Geometry: final body of the model. Coordinates: model frame, mm. Face numbers are marked on the shaded views. A direction names the side the tool comes from. Round coordinates to 2 decimals unless told otherwise and drop trailing zeros. Loops run counter-clockwise (first coordinate to the right, second up) from the corner with the lowest first, then second, coordinate; pieces in that order, holes last. Notation, with made-up numbers: (14, 14) -> (38, 14) arc R14 ccw to (38, 20) -> close; hole circle Ø9 at (83.25, 45). An arc over 180 degrees is marked (long way). Answer in a Markdown table with one row per item.
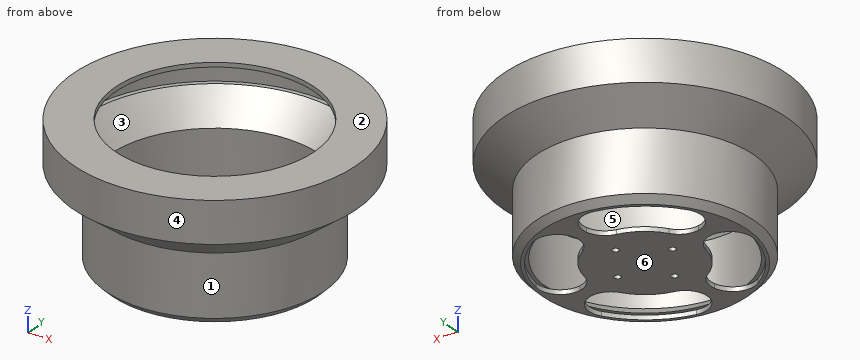
```python
from build123d import *

# Parameters (mm, degrees)
BOSS_EXTRUDE2_START = 2
SKETCH3_R           = 49.35
SKETCH3_R_2         = 1.5
BOSS_EXTRUDE2_DEPTH = 2
FILLET1_R           = 10
FILLET2_R           = 10
CHAMFER1_SIZE       = 3
SKETCH6_W           = 130.40409261
SKETCH6_H           = 9
CUT_EXTRUDE1_DEPTH  = 72
SKETCH7_R           = 64
SKETCH7_R_2         = 45
BOSS_EXTRUDE3_DEPTH = 2


with BuildPart() as part:
    # Sketch2 → Revolve1 (revolve)
    with BuildSketch(Plane(origin=(0, 0, 0), x_dir=(0, 0, -1), z_dir=(1, 0, 0)), mode=Mode.PRIVATE) as revolve1_sk:
        Polygon((65.6, 47.35), (37, 47.35), (36.023809561, 47.35), (24, 60), (24, 62), (0, 62), (0, 64), (25.567979838, 64), (37, 49.35), (65.6, 49.35), align=None)
    revolve(revolve1_sk.sketch.rotate(Axis((0, 0, 1), (0, 0, -1)), 90), axis=Axis((0, 0, 1), (0, 0, -1)))

    # Sketch3 → Boss-Extrude2 (add)
    with BuildSketch(Plane(origin=(0, 0, -65.6), x_dir=(-1, 0, 0), z_dir=(0, 0, -1)).offset(BOSS_EXTRUDE2_START)):
        with Locations(Location((0, 0, 0), (0, 0, 180))):
            Circle(SKETCH3_R)
        with Locations((-14.646406867, -3.237709975)):
            Circle(SKETCH3_R_2, mode=Mode.SUBTRACT)
        with Locations((-3.237709975, 14.646406867)):
            Circle(SKETCH3_R_2, mode=Mode.SUBTRACT)
        with Locations((3.237709975, -14.646406867)):
            Circle(SKETCH3_R_2, mode=Mode.SUBTRACT)
        with Locations((14.646406867, 3.237709975)):
            Circle(SKETCH3_R_2, mode=Mode.SUBTRACT)
        with BuildLine():
            Line((2.426668662, -24.876217196), (6.743615296, -44.404759685))
            ThreePointArc((6.743615296, -44.404759685), (-24.155488069, -37.865174318), (-43.109904177, -12.601527718))
            Line((-43.109904177, -12.601527718), (-23.581361687, -8.284581085))
            ThreePointArc((-23.581361687, -8.284581085), (-13.442501867, -21.071640807), (2.426668662, -24.876217196))
        make_face(mode=Mode.SUBTRACT)
        with BuildLine():
            Line((-24.876217196, -2.426668662), (-44.404759685, -6.743615296))
            ThreePointArc((-44.404759685, -6.743615296), (-37.865174318, 24.155488069), (-12.601527718, 43.109904177))
            Line((-12.601527718, 43.109904177), (-8.284581085, 23.581361687))
            ThreePointArc((-8.284581085, 23.581361687), (-21.071640807, 13.442501867), (-24.876217196, -2.426668662))
        make_face(mode=Mode.SUBTRACT)
        with BuildLine():
            Line((-2.426668662, 24.876217196), (-6.743615296, 44.404759685))
            ThreePointArc((-6.743615296, 44.404759685), (24.155488069, 37.865174318), (43.109904177, 12.601527718))
            Line((43.109904177, 12.601527718), (23.581361687, 8.284581085))
            ThreePointArc((23.581361687, 8.284581085), (13.442501867, 21.071640807), (-2.426668662, 24.876217196))
        make_face(mode=Mode.SUBTRACT)
        with BuildLine():
            Line((8.284581085, -23.581361687), (12.601527718, -43.109904177))
            ThreePointArc((12.601527718, -43.109904177), (37.865174318, -24.155488069), (44.404759685, 6.743615296))
            Line((44.404759685, 6.743615296), (24.876217196, 2.426668662))
            ThreePointArc((24.876217196, 2.426668662), (21.071640807, -13.442501867), (8.284581085, -23.581361687))
        make_face(mode=Mode.SUBTRACT)
    extrude(amount=-BOSS_EXTRUDE2_DEPTH)

    # Fillet1
    # the kernel refuses this fillet: 10 mm, written as the material it adds along each edge
    with BuildSketch(Plane(origin=(-12.601527718, -43.109904177, -67.6), x_dir=(-0.9040126559830293, 0.4275056933217488, 0), z_dir=(0, 0, 1))) as fillet1_piece_1:
        with BuildLine():
            CenterArc((12.508516939, -9.876472905), FILLET1_R, 80.98497739, 111.859148491)
            Line((2.758732525, -12.099467257), (0, 0))
            ThreePointArc((0, 0), (7.037725598, 0.554809366), (14.075451195, 0))
        make_face()
    extrude(amount=2)
    with BuildSketch(Plane(origin=(-8.284581085, -23.581361687, -67.6), x_dir=(-0.8924722154511289, 0.45110236604096154, 0), z_dir=(0, 0, 1))) as fillet1_piece_2:
        with BuildLine():
            CenterArc((7.785535121, 9.915423441), FILLET1_R, 194.349189504, 68.193723572)
            Line((-1.902498089, 7.437115043), (0, 0))
            ThreePointArc((0, 0), (3.243849617, 0.211393168), (6.487699233, 0))
        make_face()
    extrude(amount=2)
    with BuildSketch(Plane(origin=(-24.876217196, 2.426668662, -67.6), x_dir=(-0.9764271244734938, 0.21584733167779538, 0), z_dir=(0, 0, 1))) as fillet1_piece_3:
        with BuildLine():
            CenterArc((7.676408375, 10), FILLET1_R, 201.807483199, 68.192516801)
            ThreePointArc((-1.607964784, 6.285109014), (-0.599195502, 3.194946614), (0, 0))
            Line((0, 0), (7.676408375, 0))
        make_face()
    extrude(amount=2)
    with BuildSketch(Plane(origin=(-44.404759685, 6.743615296, -67.6), x_dir=(0.006629845184633897, -0.999978022334905, 0), z_dir=(0, 0, 1))) as fillet1_piece_4:
        with BuildLine():
            CenterArc((12.508734152, 9.876468588), FILLET1_R, 167.15489194, 111.860288522)
            Line((2.758987847, 12.099630073), (0, 0))
            ThreePointArc((0, 0), (7.037847809, -0.554828755), (14.075695618, 0))
        make_face()
    extrude(amount=2)

    # Fillet2
    # the kernel refuses this fillet: 10 mm, written as the material it adds along each edge
    with BuildSketch(Plane(origin=(-43.109904177, 12.601527718, -67.6), x_dir=(0.4275056933217496, 0.9040126559830289, 0), z_dir=(0, 0, 1))) as fillet2_piece_1:
        with BuildLine():
            CenterArc((12.508516939, -9.876472905), FILLET2_R, 80.98497739, 111.859148491)
            Line((2.758732525, -12.099467257), (0, 0))
            ThreePointArc((0, 0), (7.037725598, 0.554809366), (14.075451195, 0))
        make_face()
    extrude(amount=2)
    with BuildSketch(Plane(origin=(-23.581361687, 8.284581085, -67.6), x_dir=(-0.9764271244734907, 0.21584733167780967, 0), z_dir=(0, 0, 1)), Plane(origin=(8.284581085, 23.581361687, -67.6), x_dir=(0.21584733167780917, 0.9764271244734908, 0), z_dir=(0, 0, 1)), Plane(origin=(23.581361687, -8.284581085, -67.6), x_dir=(0.9764271244734907, -0.21584733167780934, 0), z_dir=(0, 0, 1))) as fillet2_piece_2:
        with BuildLine():
            CenterArc((7.676599451, -10), FILLET2_R, 90, 68.193723572)
            ThreePointArc((-1.607851949, -6.285304563), (-0.599127572, -3.195042028), (0, 0))
            Line((0, 0), (7.676599451, 0))
        make_face()
    extrude(amount=2)
    with BuildSketch(Plane(origin=(2.426668662, 24.876217196, -67.6), x_dir=(0.2158473316777956, 0.9764271244734938, 0), z_dir=(0, 0, 1))) as fillet2_piece_3:
        with BuildLine():
            CenterArc((7.676408375, 10), FILLET2_R, 201.807483199, 68.192516801)
            ThreePointArc((-1.607964784, 6.285109014), (-0.599195502, 3.194946614), (0, 0))
            Line((0, 0), (7.676408375, 0))
        make_face()
    extrude(amount=2)
    with BuildSketch(Plane(origin=(6.743615296, 44.404759685, -67.6), x_dir=(-0.999978022334905, -0.006629845184635393, 0), z_dir=(0, 0, 1)), Plane(origin=(44.404759685, -6.743615296, -67.6), x_dir=(-0.006629845184635893, 0.999978022334905, 0), z_dir=(0, 0, 1)), Plane(origin=(-6.743615296, -44.404759685, -67.6), x_dir=(0.999978022334905, 0.00662984518463539, 0), z_dir=(0, 0, 1))) as fillet2_piece_4:
        with BuildLine():
            CenterArc((12.508734152, 9.876468588), FILLET2_R, 167.15489194, 111.860288522)
            Line((2.758987847, 12.099630073), (0, 0))
            ThreePointArc((0, 0), (7.037847809, -0.554828755), (14.075695618, 0))
        make_face()
    extrude(amount=2)
    with BuildSketch(Plane(origin=(24.876217196, -2.426668662, -67.6), x_dir=(-0.032899449429987265, 0.9994586665926729, 0), z_dir=(0, 0, 1)), Plane(origin=(-2.426668662, -24.876217196, -67.6), x_dir=(0.9994586665926729, 0.03289944942998876, 0), z_dir=(0, 0, 1))) as fillet2_piece_5:
        with BuildLine():
            CenterArc((7.785341334, -9.915427669), FILLET2_R, 97.456900257, 68.192516801)
            Line((-1.902631601, -7.436883658), (0, 0))
            ThreePointArc((0, 0), (3.243768875, -0.2113826), (6.48753775, 0))
        make_face()
    extrude(amount=2)
    with BuildSketch(Plane(origin=(12.601527718, 43.109904177, -67.6), x_dir=(-0.21584733167780898, -0.9764271244734908, 0), z_dir=(0, 0, 1)), Plane(origin=(43.109904177, -12.601527718, -67.6), x_dir=(-0.9764271244734909, 0.21584733167780892, 0), z_dir=(0, 0, 1))) as fillet2_piece_6:
        with BuildLine():
            CenterArc((12.40998441, 10), FILLET2_R, 158.140851509, 111.859148491)
            ThreePointArc((3.128964851, 13.723261468), (1.023555255, 6.984964542), (0, 0))
            Line((0, 0), (12.40998441, 0))
        make_face()
    extrude(amount=2)

    # Sketch5 → Revolve2 (revolve)
    with BuildSketch(Plane(origin=(0, 0, 0), x_dir=(1, 0, 0), z_dir=(0, 1, 0)), mode=Mode.PRIVATE) as revolve2_sk:
        Polygon((-47.35, 61.6), (-43.35, 65.6), (-47.35, 65.6), align=None)
    revolve(revolve2_sk.sketch.rotate(Axis((0, 0, 0), (0, 0, -1)), 180), axis=Axis((0, 0, 0), (0, 0, -1)))

    # Chamfer1
    chamfer1_edges = [part.edges().sort_by_distance(p)[0] for p in [
        (-49.35, 0, -67.6),
    ]]
    chamfer(chamfer1_edges, length=CHAMFER1_SIZE)

    # Sketch6 → Cut-Extrude1 (cut, symmetric)
    with BuildSketch(Plane(origin=(0, 0, 0), x_dir=(1, 0, 0), z_dir=(0, 1, 0))):
        with Locations((-1.202046305, 4.5)):
            Rectangle(SKETCH6_W, SKETCH6_H)
    extrude(amount=CUT_EXTRUDE1_DEPTH, both=True, mode=Mode.SUBTRACT)

    # Sketch7 → Boss-Extrude3 (add)
    with BuildSketch(Plane.XY.offset(-9)):
        Circle(SKETCH7_R)
        Circle(SKETCH7_R_2, mode=Mode.SUBTRACT)
    extrude(amount=BOSS_EXTRUDE3_DEPTH)


solid = part.part
```
Item 1: Cut plane A-A (z = -60). Output: boundary loops of the cut face in (x, y), then the cut area to 3 significant figures.
Answer:
| item | result |
|---|---|
| outline | circle Ø98.7 at (0, 0); hole circle Ø94.7 at (0, 0) |
| area | 608 mm² |
Item 2: Reachability of the marked faces 1, 2 and 3 from +Z, -Z, +X, -X, +Y, -Y: full face, straight path, thin tool, end or side. Return the list, or none.
Answer:
| item | result |
|---|---|
| face 1 | -Z |
| face 2 | +Z, +X, -X, +Y, -Y |
| face 3 | none |
Item 3: Draft query along Z for the marked faces 4, 5 and 6. Return one class per face: pulls with the +Z half, pulls with the -Z half, needs draft (parallel to the pull), parting line crosses it, or undercut.
Answer:
| item | result |
|---|---|
| face 4 | needs draft |
| face 5 | undercut |
| face 6 | pulls with the -Z half |
Item 4: Pin query (flat end, axial travel): pin 1 Ø5 at (x, y) = (3.24, 14.65) entering from -Z; pin 2 Ø4 at (x, z) = (-20, -39.5) entering from +Y; pin 3 Ø3 at (x, z) = (-4, -14) entering from -Y; pin 4 Ø1.5 at (x, z) = (-10.5, -13.5) entering from +Y. Return the tip coordinate at first contact, or that it passes through.
Answer:
| item | result |
|---|---|
| pin 1 | stops at z = -67.6 |
| pin 2 | stops at y = 45.95 |
| pin 3 | stops at y = -63.95 |
| pin 4 | stops at y = 63.25 |
Item 5: Cut plane B-B (y = -29.5). Count the separate pieces of the cut face and the enclosed holes in it, then the cut area to 3 significant figures.
Answer:
| item | result |
|---|---|
| separate pieces | 3 |
| enclosed holes | 0 |
| area | 483 mm² |
Item 6: Line query: probe 1 along Y at (x, z) = (0, -8); probe 2 along Y at (x, z) = (0, -21); probe 3 along Z at (x, y) = (-39, 14.5). Output: solid intervals per line, ascending. Write a range as [from, to].
Answer:
| item | result |
|---|---|
| probe 1 | y = [-64, -45], [45, 64] |
| probe 2 | y = [-64, -62], [62, 64] |
| probe 3 | z = [-67.6, -65.6] |
Item 7: Cut plane D-D (z = -16.5). Output: boundary loops of the cut face in (x, y), then the cut area to 3 significant figures.
Answer:
| item | result |
|---|---|
| outline | circle Ø128 at (0, 0); hole circle Ø124 at (0, 0) |
| area | 792 mm² |
